Could you check a few things on this model? Use its own coordinates, in mm. A direction names the side the tool comes from. Give positions to 0.01 mm unless a question says otherwise; leave off trailing zeros. Write each loop counter-clockwise with the first axis right and the second up, starting at its lowest first coordinate (ties: lowest second). Pieces come first, ordered by that corner, then holes. Notation, with made-up numbers: (-22.5, 10) - (34.5, 10) arc R24 cw to (34.5, 24) - close; hole circle Ø11 at (17, 18). An arc over 180 degrees is marked (long way). Answer in a Markdown table with one row per item.
from build123d import *
from OCP.BRepFilletAPI import BRepFilletAPI_MakeChamfer

# Parameters (mm, degrees)
BOSS_EXTRUDE1_DEPTH = 4.5
CUT_EXTRUDE1_DEPTH  = 43.429353047
SKETCH3_W           = 4.25
SKETCH3_H           = 5
CUT_EXTRUDE2_DEPTH  = 43.429353047
SKETCH4_R           = 1.5
CUT_EXTRUDE3_DEPTH  = 43.429353047
BOSS_EXTRUDE2_DEPTH = 4.5
CHAMFER1_SIZE       = 2
CHAMFER1_SIZE2      = 0.535898385
CHAMFER2_SIZE       = 2
SKETCH8_R           = 0.125
CUT_EXTRUDE4_DEPTH  = 48.236770635


with BuildPart() as part:
    # Sketch1 → Boss-Extrude1 (new body)
    with BuildSketch(Plane(origin=(0, 0, 0), x_dir=(1, 0, 0), z_dir=(0, 1, 0))):
        Polygon((-18.5, -18.5), (0, 0), (36, 0), (36, -22), (-18.5, -22), align=None)
    extrude(amount=BOSS_EXTRUDE1_DEPTH)

    # Sketch2 → Cut-Extrude1 (cut, through all)
    with BuildSketch(Plane(origin=(0, 4.5, 0), x_dir=(1, 0, 0), z_dir=(0, 1, 0))):
        Polygon((-6.363961031, -9.192388155), (-2.828427125, -5.656854249), (-0.707106781, -7.778174593), (-4.242640687, -11.313708499), align=None)
        Polygon((-10.960155108, -13.788582233), (-8.838834765, -15.909902577), (-12.374368671, -19.445436483), (-14.495689014, -17.324116139), align=None)
    cut_extrude1 = extrude(amount=-CUT_EXTRUDE1_DEPTH, mode=Mode.SUBTRACT)

    # Mirror1: Cut-Extrude1 across plane
    add(cut_extrude1.mirror(Plane(origin=(0, 0, 0), x_dir=(0, 0, 1), z_dir=(1, 0, 0))), mode=Mode.SUBTRACT)

    # Sketch3 → Cut-Extrude2 (cut, through all)
    with BuildSketch(Plane(origin=(0, 4.5, 0), x_dir=(1, 0, 0), z_dir=(0, 1, 0))):
        with Locations((30.875, -4.5)):
            Rectangle(SKETCH3_W, SKETCH3_H)
        with Locations((30.875, -17.5)):
            Rectangle(SKETCH3_W, SKETCH3_H)
    extrude(amount=-CUT_EXTRUDE2_DEPTH, mode=Mode.SUBTRACT)

    # Sketch4 → Cut-Extrude3 (cut, through all)
    with BuildSketch(Plane(origin=(0, 4.5, 0), x_dir=(1, 0, 0), z_dir=(0, 1, 0))):
        with Locations(Location((0, -18, 0), (0, 0, 270))):
            Circle(SKETCH4_R)
        with Locations(Location((25, -3, 0), (0, 0, 270))):
            Circle(SKETCH4_R)
    extrude(amount=-CUT_EXTRUDE3_DEPTH, mode=Mode.SUBTRACT)

    # Sketch5 → Boss-Extrude2 (add)
    with BuildSketch(Plane(origin=(0, 4.5, 0), x_dir=(1, 0, 0), z_dir=(0, 1, 0))):
        Polygon((-5, -22), (5, -22), (5, -26.25), (10, -26.25), (10, -30.25), (-10, -30.25), (-10, -26.25), (-5, -26.25), align=None)
    extrude(amount=-BOSS_EXTRUDE2_DEPTH)

    # Chamfer1: one chamfer whose edges measure the first distance from different faces: ONE call of the kernel's chamfer builder (chamfer() names one face for all edges)
    chamfer1_edges_1 = [part.edges().sort_by_distance(p)[0] for p in [
        (-10, 2.25, 26.25),
    ]]
    chamfer1_side_1 = [part.faces().sort_by_distance(p)[0] for p in [
        (-7.5, 2.25, 26.25),
    ]]
    chamfer1_edges_2 = [part.edges().sort_by_distance(p)[0] for p in [
        (10, 2.25, 26.25),
    ]]
    chamfer1_side_2 = [part.faces().sort_by_distance(p)[0] for p in [
        (7.5, 2.25, 26.25),
    ]]
    chamfer1 = BRepFilletAPI_MakeChamfer(part.part.solid().wrapped)
    for e in chamfer1_edges_1:
        chamfer1.Add(CHAMFER1_SIZE, CHAMFER1_SIZE2, e.wrapped, chamfer1_side_1[0].wrapped)  # the first distance lies on this face
    for e in chamfer1_edges_2:
        chamfer1.Add(CHAMFER1_SIZE, CHAMFER1_SIZE2, e.wrapped, chamfer1_side_2[0].wrapped)  # the first distance lies on this face
    add(Compound.cast(chamfer1.Shape()), mode=Mode.REPLACE)

    # Chamfer2
    chamfer2_edges = [part.edges().sort_by_distance(p)[0] for p in [
        (36, 2.25, 0),
        (36, 2.25, 22),
    ]]
    chamfer(chamfer2_edges, length=CHAMFER2_SIZE)

    # Sketch8 → Cut-Extrude4 (cut, through all)
    with BuildSketch(Plane(origin=(0, 4.5, 0), x_dir=(1, 0, 0), z_dir=(0, 1, 0))):
        with Locations((-12.374368671, -19.445436483)):
            Circle(SKETCH8_R)
    cut_extrude4 = extrude(amount=-CUT_EXTRUDE4_DEPTH, mode=Mode.SUBTRACT)

    # Sketch-Pattern1: Cut-Extrude4 at 27 more places
    with Locations((-2.12132, 0, -2.12132), (1.414214, 0, -5.656854), (3.535534, 0, -3.535534), (8.131728, 0, -8.131728), (6.010408, 0, -10.253048), (9.545942, 0, -13.788582), (11.667262, 0, -11.667262), (13.081475, 0, -11.667262), (15.202796, 0, -13.788582), (18.73833, 0, -10.253048), (16.617009, 0, -8.131728), (23.334524, 0, -5.656854), (21.213203, 0, -3.535534), (24.748737, 0, 0), (26.870058, 0, -2.12132), (41.124369, 0, -12.445436), (41.124369, 0, -17.445436), (45.374369, 0, -17.445436), (45.374369, 0, -12.445436), (45.374369, 0, -4.445436), (41.124369, 0, -4.445436), (41.124369, 0, 0.554564), (45.374369, 0, 0.554564), (17.374369, 0, 6.804564), (7.374369, 0, 6.804564), (7.374369, 0, 2.554564), (17.374369, 0, 2.554564)):
        add(cut_extrude4, mode=Mode.SUBTRACT)


solid = part.part
1) Imagine slicing it at C-C (y = 3.7). State how many separate pieces and enclosed holes the cut face has, then the cut area to 3 significant figures.
Check values:
| item | result |
|---|---|
| separate pieces | 1 |
| enclosed holes | 8 |
| area | 1,030 mm2 |
2) Imagine slicing it at A-A (x = -7). List the corners of the cut face in (y, z) for me.
Check values:
| item | result |
|---|---|
| outline | (0, 7) - (4.5, 7) - (4.5, 22) - (0, 22) - close; (0, 26.25) - (4.5, 26.25) - (4.5, 30.25) - (0, 30.25) - close |
3) On a 3-axis mill with a long thin cutter (end or side, diameter ignored), from which of +Z, -Z, +X, -X, +Y, -Y can I reach the whole of each face in a straight line? I mean faces 5 (the face through (7, 2, 26.25)), 6 (the face through (10, 2, 28)), 7 (the face through (31, 2, 7)), 8 (the face through (-5, 2, 24)). Say none if no direction works.
Check values:
| item | result |
|---|---|
| face 5 | +X, +Y, -Y |
| face 6 | +Z, +X, +Y, -Y |
| face 7 | +Y, -Y |
| face 8 | -X, +Y, -Y |
4) If I drill on line 1 (X direction, y = 3.25, z = 10.5); line 2 (X direction, y = 1.55, z = 18); line 3 (Z direction, x = 30.5, y = 3.45), over which ranges is the centre line in solid material (lowest first)?
Check values:
| item | result |
|---|---|
| line 1 | x = -10.5 to -5.06, -3.43 to 3.43, 5.06 to 36 |
| line 2 | x = -18 to -13.82, -10.93 to -1.5, 1.5 to 10.93, 13.82 to 28.75, 33 to 36 |
| line 3 | z = 0 to 2, 7 to 15, 20 to 22 |
5) We'd pull the mould along Z, two halves only. Please class faces 1 (the face through (-9, 2, 9)), 2 (the face through (9, 4.5, 15)), 3 (the face through (9.91, 2.28, 14.84)), 4 (the face through (12.75, 2.28, 15.58)): +Z half, -Z half, draft (parallel to the pull), parting line (faces both ways), or undercut.
Check values:
| item | result |
|---|---|
| face 1 | -Z half |
| face 2 | draft |
| face 3 | undercut |
| face 4 | undercut |
6) Will these pins go through, and if not, where does the flat tip stop? P1, Ø0.9, axis at x = -6, y = 1.5, coming from the -Z side; P2, Ø2, axis at x = 32, y = 2, coming from the +Z side; P3, Ø1, axis at y = 3, z = 4, coming from the -X side.
Check values:
| item | result |
|---|---|
| P1 | stops at z = 5.55 |
| P2 | stops at z = 22 |
| P3 | stops at x = -4.5 |
7) Imagine slicing it at B-B (z = 18). List the corners of the cut face in (x, y) for me.
Check values:
| item | result |
|---|---|
| outline | (-18, 0) - (-13.82, 0) - (-13.82, 4.5) - (-18, 4.5) - close; (-10.93, 0) - (-1.5, 0) - (-1.5, 4.5) - (-10.93, 4.5) - close; (1.5, 0) - (10.93, 0) - (10.93, 4.5) - (1.5, 4.5) - close; (13.82, 0) - (28.75, 0) - (28.75, 4.5) - (13.82, 4.5) - close; (33, 0) - (36, 0) - (36, 4.5) - (33, 4.5) - close |
8) Imagine slicing it at D-D (x = -13.5). List the corners of the cut face in (y, z) for me.
Check values:
| item | result |
|---|---|
| outline | (0, 13.5) - (4.5, 13.5) - (4.5, 16.33) - (0, 16.33) - close; (0, 18.32) - (4.5, 18.32) - (4.5, 22) - (0, 22) - close |
